from build123d import *

# Parameters (mm, degrees)
SKETCH1_R               = 7.5
BOSS_EXTRUDE1_DEPTH     = 8
CROQUIS6_W              = 20
CROQUIS6_H              = 20
SALIENTE_EXTRUIR5_DEPTH = 11
CROQUIS7_R              = 1.5
CORTAR_EXTRUIR1_DEPTH   = 10


with BuildPart() as part:
    # Sketch1 → Boss-Extrude1 (new body)
    with BuildSketch(Plane(origin=(0, 0, 0), x_dir=(1, 0, 0), z_dir=(0, 1, 0))):
        with BuildLine():
            Line((50.606601718, 10.606601718), (50.606601718, 0))
            Line((50.606601718, 0), (70.606601718, 0))
            Line((70.606601718, 0), (70.606601718, 10.606601718))
            ThreePointArc((70.606601718, 10.606601718), (53.033008589, 53.033008589), (10.606601718, 70.606601718))
            Line((10.606601718, 70.606601718), (-9.393398282, 70.606601718))
            Line((-9.393398282, 70.606601718), (-9.393398282, 50.606601718))
            Line((-9.393398282, 50.606601718), (10.606601718, 50.606601718))
            ThreePointArc((10.606601718, 50.606601718), (38.890872965, 38.890872965), (50.606601718, 10.606601718))
        make_face()
        with Locations(Location((60.606601718, 10.606601718, 0), (0, 0, 270))):
            Circle(SKETCH1_R, mode=Mode.SUBTRACT)
    extrude(amount=BOSS_EXTRUDE1_DEPTH)

    # Croquis6 → Saliente-Extruir5 (add)
    with BuildSketch(Plane.XZ):
        with Locations((0.606601718, -60.606601718)):
            Rectangle(CROQUIS6_W, CROQUIS6_H)
    extrude(amount=SALIENTE_EXTRUIR5_DEPTH)

    # Croquis7 → Cortar-Extruir1 (cut)
    with BuildSketch(Plane.XZ.offset(11)):
        with Locations(Location((-5.393398282, -60.606601718, 0), (0, 0, 270))):
            Circle(CROQUIS7_R)
        with Locations(Location((6.606601718, -60.606601718, 0), (0, 0, 90))):
            Circle(CROQUIS7_R)
        with Locations(Location((0.606601718, -66.606601718, 0), (0, 0, 270))):
            Circle(CROQUIS7_R)
        with Locations(Location((0.606601718, -54.606601718, 0), (0, 0, 90))):
            Circle(CROQUIS7_R)
    extrude(amount=-CORTAR_EXTRUIR1_DEPTH, mode=Mode.SUBTRACT)


solid = part.part
Check sheet for the modelled part. Datum: model origin and axes. Units: mm. A direction names the side the tool comes from. Give positions to 0.01 mm unless a question says otherwise; leave off trailing zeros. Loops run counter-clockwise (first coordinate to the right, second up) from the corner with the lowest first, then second, coordinate; pieces in that order, holes last. Notation, with made-up numbers: M 87,56.25 L 118,56.25 A26 ccw 118,84.25 Z; hole C -26,73.5 d9. An arc over 180 degrees is marked long. Answer as a JSON object with one key per item and string values. Group by question number.
Q1. Access from +Z, -Z, +X, -X, +Y, -Y to the whole of each face (thin tool, end or side, straight path). Record for faces 5 (the flat face through (40, 0, -44)), 6 (the flat face through (0, -1, -50.607)), 7 (the flat face through (1, -1, -67)).
Q2. Cross-section at C-C on z = -52. Record the cut outline in (x, y), then the cut area to 3 significant figures.
Q3. Cross-section at B-B on y = -7. Record the cut outline in (x, z), then the cut area to 3 significant figures.
Q4. Go/stop test with flat-tipped pins: P1, Ø1.5, axis at x = -1, y = 5, coming from the +Z side; P2, Ø1.8, axis at x = 0.61, z = -54.61, coming from the -Y side; P3, Ø2.5, axis at x = 1, z = -66.5, coming from the -Y side; P4, Ø8, axis at x = 31.5, y = -6, coming from the +Z side. Record where each tip stops, or that it passes through.
Q5. Cross-section at D-D on x = 46. Record the cut outline in (y, z), then the cut area to 3 significant figures.
Q6. Cross-section at A-A on y = 1.75. Record the cut outline in (x, z), then the cut area to 3 significant figures.
Q7. Material ranges on line 1 along Z through (x, y) = (10, -8.75); line 2 along Y through (x, z) = (50.5, -33); line 3 along Z through (x, y) = (-5, -1.25), recorded low to high. Write a range as [from, to].
Q8. Release check for a two-part mould opening along X. For faces 1 (the flat face through (50.607, 4, -5)), 2 (the flat face through (0, -1, -70.607)), 3 (the flat face through (10.607, -5, -61)), 4 (the cylindrical face through (0.673, -6.07, -65.108)) record: released by +X, released by -X, zero draft, split by the parting line, or undercut.
Evaluation:
{
 "1": {"face 5": "+Z, -Z, +X, -Y", "face 6": "+Z, -X, +Y, -Y", "face 7": "-Y"},
 "2": {"outline": "M -9.39,-11 L 10.61,-11 L 10.61,0 L 54.04,0 L 54.04,8 L -9.39,8 Z", "area": "727 mm2"},
 "3": {"outline": "M -9.39,-70.61 L 10.61,-70.61 L 10.61,-50.61 L -9.39,-50.61 Z; hole C -5.39,-60.61 d3; hole C 0.61,-66.61 d3; hole C 0.61,-54.61 d3; hole C 6.61,-60.61 d3", "area": "372 mm2"},
 "4": {"P1": "stops at z = -50.61", "P2": "stops at y = -1", "P3": "stops at y = -11", "P4": "passes through"},
 "5": {"outline": "M 0,-59.06 L 8,-59.06 L 8,-29.24 L 0,-29.24 Z", "area": "239 mm2"},
 "6": {"outline": "M -9.39,-70.61 L 10.61,-70.61 A60 ccw 70.61,-10.61 L 70.61,0 L 50.61,0 L 50.61,-10.61 A40 cw 10.61,-50.61 L -9.39,-50.61 Z; hole C 60.61,-10.61 d15", "area": "2,010 mm2"},
 "7": {"line 1": "z = [-70.61, -50.61]", "line 2": "y = [0, 8]", "line 3": "z = [-70.61, -62.05], [-59.16, -50.61]"},
 "8": {"face 1": "released by -X", "face 2": "zero draft", "face 3": "released by +X", "face 4": "undercut"}
}
